from build123d import *

# Parameters (mm, degrees)
SKETCH1_R           = 44.45
BOSS_EXTRUDE1_DEPTH = 3.81
SKETCH2_R           = 38.4429
SKETCH2_R_2         = 34.6329
BOSS_EXTRUDE2_DEPTH = 12.7
FILLET1_R           = 1.27
SKETCH4_R           = 6.0833
CUT_EXTRUDE1_DEPTH  = 17.51


with BuildPart() as part:
    # Sketch1 → Boss-Extrude1 (new body)
    with BuildSketch(Plane.XY):
        Circle(SKETCH1_R)
    extrude(amount=BOSS_EXTRUDE1_DEPTH)

    # Sketch2 → Boss-Extrude2 (add)
    with BuildSketch(Plane(origin=(0, 0, 0), x_dir=(-1, 0, 0), z_dir=(0, 0, -1))):
        Circle(SKETCH2_R)
        Circle(SKETCH2_R_2, mode=Mode.SUBTRACT)
    extrude(amount=BOSS_EXTRUDE2_DEPTH)

    # Fillet1
    fillet1_edges = [part.edges().sort_by_distance(p)[0] for p in [
        (-44.45, 0, 3.81),
        (38.4429, 0, -12.7),
        (34.6329, 0, 0),
        (34.6329, 0, -12.7),
    ]]
    fillet(fillet1_edges, radius=FILLET1_R)

    # Sketch4 → Cut-Extrude1 (cut, through all)
    with BuildSketch(Plane.XY.offset(3.81)):
        with Locations((0, 24.5999)):
            Circle(SKETCH4_R)
    extrude(amount=-CUT_EXTRUDE1_DEPTH, mode=Mode.SUBTRACT)


solid = part.part
CAD build for the part. Positions are in the model's coordinates, mm. A direction names the side the tool comes from. Round coordinates to 2 decimals unless told otherwise and drop trailing zeros. Write each loop counter-clockwise with the first axis right and the second up, starting at its lowest first coordinate (ties: lowest second). Pieces come first, ordered by that corner, then holes. Notation, with made-up numbers: M 81.5,-28.75 L 108.5,-28.75 A12 ccw 108.5,-24.75 Z; hole C 73.25,51.25 d5. An arc over 180 degrees is marked long. Put each result on its own line as item: value. Start each with the question number.
1) Pin check, flat tips, straight feed: pin 1 Ø10 at (x, y) = (16.5, 14) entering from -Z; pin 2 Ø8 at (y, z) = (8, 2) entering from -X; pin 3 Ø5 at (y, z) = (2.5, -4.5) entering from -X. Stop position of each tip, or through.
2) Saw through at C-C, the plane z = -8.5. Write the cut outline in (x, y), and give its area (3 significant figures).
3) Drill centre lines: probe 1 along X at (y, z) = (1, -10.25); probe 2 along Y at (x, z) = (0, 1.6); probe 3 along Z at (x, y) = (1, 9). Where is each one in solid material? Low to high. Write a range as [from, to].
4) 3-axis set-ups, long thin cutter, end or side, ignore diameter. For faces 1 (the flat face through (-1, 1, 3.81)), 2 (the cylindrical face through (-17.739, -34.105, -5.635)): which of +Z, -Z, +X, -X, +Y, -Y reach the whole face in a straight line?
5) Saw through at B-B, the plane y = 0. Write the cut outline in (x, z), and give its area (3 significant figures).
6) Pull direction Y, two halves, no side cores. Call faces 3 (the cylindrical face through (-0.79, 30.63, 1.93)), 4 (the cylindrical face through (42.397, 13.352, 1.252)), 5 (the flat face through (19.4, 30.5, -12.7)): pulls with the +Y half, pulls with the -Y half, needs draft (parallel to the pull), parting line crosses it, or undercut.
7) Saw through at A-A, the plane x = 0. Write the cut outline in (y, z), and give its area (3 significant figures).
Resolved:
1. pin 1: z = 0
1. pin 2: x = -44.27
1. pin 3: x = -38.44
2. outline: C 0,0 d76.89; hole C 0,0 d69.27
2. area: 875 mm²
3. probe 1: [-38.43, -34.62], [34.62, 38.43]
3. probe 2: [-44.45, 18.52], [30.68, 44.45]
3. probe 3: [0, 3.81]
4. face 1: +Z, +X, -X, +Y, -Y
4. face 2: -Z
5. outline: M -44.45,0 L -38.44,0 L -38.44,-11.43 A1.27 ccw -37.17,-12.7 L -35.9,-12.7 A1.27 ccw -34.63,-11.43 L -34.63,-1.27 A1.27 cw -33.36,0 L 33.36,0 A1.27 cw 34.63,-1.27 L 34.63,-11.43 A1.27 ccw 35.9,-12.7 L 37.17,-12.7 A1.27 ccw 38.44,-11.43 L 38.44,0 L 44.45,0 L 44.45,2.54 A1.27 ccw 43.18,3.81 L -43.18,3.81 A1.27 ccw -44.45,2.54 Z
5. area: 434 mm²
6. face 3: undercut
6. face 4: parting line crosses it
6. face 5: needs draft
7. outline: M -44.45,0 L -38.44,0 L -38.44,-11.43 A1.27 ccw -37.17,-12.7 L -35.9,-12.7 A1.27 ccw -34.63,-11.43 L -34.63,-1.27 A1.27 cw -33.36,0 L 18.52,0 L 18.52,3.81 L -43.18,3.81 A1.27 ccw -44.45,2.54 Z; M 30.68,0 L 33.36,0 A1.27 cw 34.63,-1.27 L 34.63,-11.43 A1.27 ccw 35.9,-12.7 L 37.17,-12.7 A1.27 ccw 38.44,-11.43 L 38.44,0 L 44.45,0 L 44.45,2.54 A1.27 ccw 43.18,3.81 L 30.68,3.81 Z
7. area: 388 mm²
